from build123d import *

# Parameters (mm, degrees)
SKETCH1_R           = 25
BOSS_EXTRUDE1_DEPTH = 1
SKETCH2_R           = 4
CUT_EXTRUDE1_DEPTH  = 1


with BuildPart() as part:
    # Sketch1 → Boss-Extrude1 (new body)
    with BuildSketch(Plane(origin=(0, 0, 0), x_dir=(1, 0, 0), z_dir=(0, 1, 0))):
        Circle(SKETCH1_R)
    extrude(amount=BOSS_EXTRUDE1_DEPTH)

    # Sketch2 → Cut-Extrude1 (cut)
    with BuildSketch(Plane(origin=(0, 1, 0), x_dir=(1, 0, 0), z_dir=(0, 1, 0))):
        with Locations((0, 12.5)):
            Circle(SKETCH2_R)
        with Locations((12.5, 0)):
            Circle(SKETCH2_R)
        with Locations((-12.5, 0)):
            Circle(SKETCH2_R)
        with Locations((0, -12.5)):
            Circle(SKETCH2_R)
    extrude(amount=-CUT_EXTRUDE1_DEPTH, mode=Mode.SUBTRACT)


solid = part.part
Check sheet for the modelled part. Datum: model origin and axes. Units: mm. Round coordinates to 2 decimals unless told otherwise and drop trailing zeros. Loops run counter-clockwise (first coordinate to the right, second up) from the corner with the lowest first, then second, coordinate; pieces in that order, holes last. Notation, with made-up numbers: M -21.75,13 L -17.75,13 A20 ccw -17.75,36 Z; hole C -4,10.25 d6. An arc over 180 degrees is marked long. One line per item, written item: value.
(1) Sectioned sample at A-A, the plane x = 0. Record the cut outline in (y, z), then the cut area to 3 significant figures.
Computed values:
outline: M 0,-25 L 1,-25 L 1,-16.5 L 0,-16.5 Z; M 0,-8.5 L 1,-8.5 L 1,8.5 L 0,8.5 Z; M 0,16.5 L 1,16.5 L 1,25 L 0,25 Z
area: 34.0 mm^2
(2) Sectioned sample at C-C, the plane z = -1.5. Record the cut outline in (x, y).
Computed values:
outline: M -24.95,0 L -16.21,0 L -16.21,1 L -24.95,1 Z; M -8.79,0 L 8.79,0 L 8.79,1 L -8.79,1 Z; M 16.21,0 L 24.95,0 L 24.95,1 L 16.21,1 Z
(3) Sectioned sample at D-D, the plane x = 12.5. Record the cut outline in (y, z).
Computed values:
outline: M 0,-21.65 L 1,-21.65 L 1,-4 L 0,-4 Z; M 0,4 L 1,4 L 1,21.65 L 0,21.65 Z
(4) Sectioned sample at B-B, the plane y = 0.5. Record the cut outline in (x, z).
Computed values:
outline: C 0,0 d50; hole C -12.5,0 d8; hole C 0,-12.5 d8; hole C 0,12.5 d8; hole C 12.5,0 d8
(5) Thickness scan on line 1 (Z direction, x = 0, y = 0.65); line 2 (X direction, y = 0.7, z = -2). Record the ranges inside material, lowest first.
Computed values:
line 1: z = -25 to -16.5, -8.5 to 8.5, 16.5 to 25
line 2: x = -24.92 to -15.96, -9.04 to 9.04, 15.96 to 24.92
(6) Depth check by flat-ended pin: pin 1 Ø7 at (x, z) = (0, 12.5) entering from +Y (1 decimal). Enter the tip coordinate at first touch or a pass-through.
Computed values:
pin 1: passes through
(7) Release check for a two-part mould opening along Z. For faces 1 (the face through (0, 0, 0)), 2 (the face through (23.846, 0.493, -7.509)), 3 (the face through (-0.521, 0.507, -16.466)) record: +Z half, -Z half, draft (parallel to the pull), parting line (faces both ways), or undercut.
Computed values:
face 1: draft
face 2: parting line
face 3: undercut
